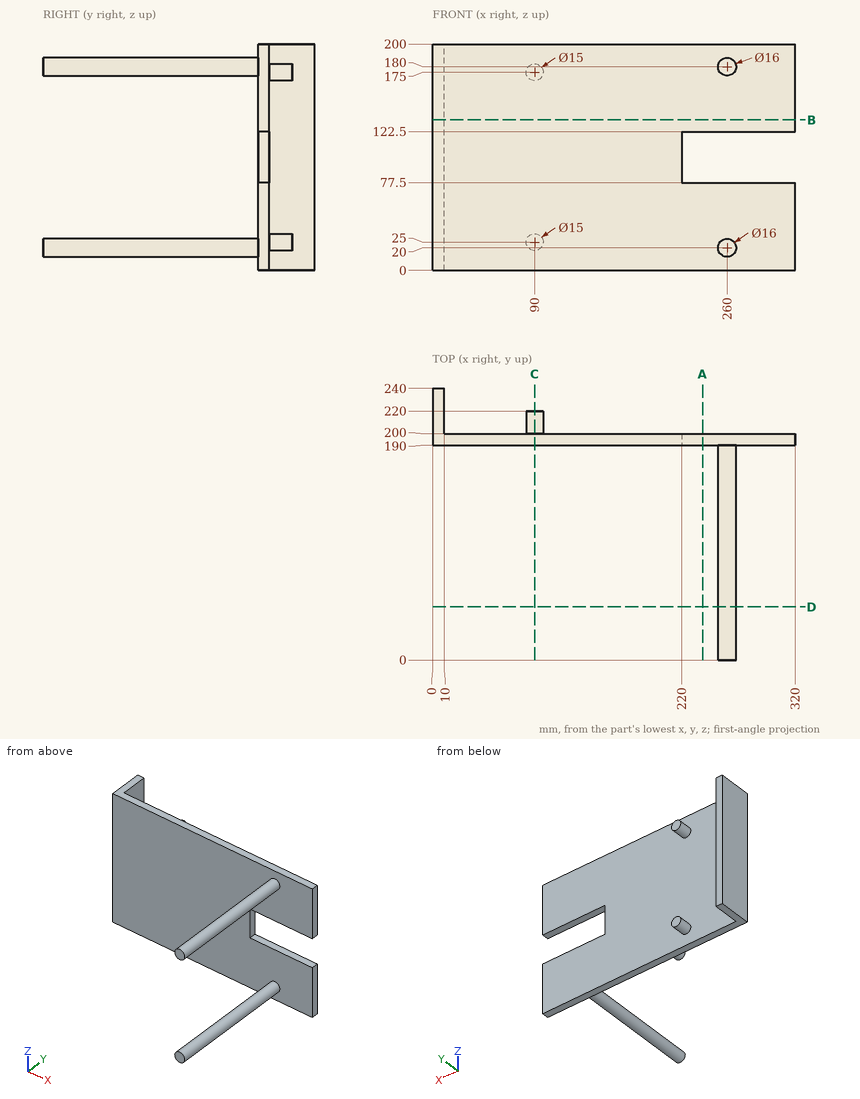
Can you work these out from the drawing? Everything is in mm from the part's minimum corner. Give positions to 0.01 mm unless a question says otherwise; leave off trailing zeros. Order: outer loops, then holes, each group sorted by start corner. A loop starts at its lowest first (then second) coordinate and runs counter-clockwise, first axis right, second up. Notation, with made-up numbers: M 82,32 L 137,32 A25 cw 137,71 Z; hole C 39,54.25 d10. An arc over 180 degrees is marked long. Use a Markdown table: item, result. Add a question column.
Item 1: Suppose I cut it at D-D (y = 47). List the corners of the cut face in (x, z) for me, then the cut area to 3 significant figures.
Item 2: Suppose I cut it at A-A (x = 238.5). List the corners of the cut face in (y, z) for me, then the cut area to 3 significant figures.
Item 3: Suppose I cut it at B-B (z = 133). List the corners of the cut face in (x, y) for me.
Item 4: Suppose I cut it at C-C (x = 90). List the corners of the cut face in (y, z) for me.
Item 5: Will these pins go through, and if not, where does the flat tip stop? pin 1 (1.5 mm diameter, centred on x = 136, z = 87, fed in from -Y); pin 2 (4.5 mm diameter, centred on x = 90.5, z = 26.5, fed in from +Y); pin 3 (12 mm diameter, centred on y = 213.5, z = 127.5, fed in from +X); pin 4 (8 mm diameter, centred on x = 251, y = 197.5, fed in from -Z).
Item 6: If I drill on L1, parallel to X at y = 223, z = 174.5; L2, parallel to Y at x = 188, z = 126; L3, parallel to X at y = 55, z = 21.5, over which ranges is the centre line in solid material (lowest first)? Write a range as [from, to].
Answer sheet:
| question | item | result |
|---|---|---|
| 1 | outline | C 260,20 d16; C 260,180 d16 |
| 1 | area | 402 mm² |
| 2 | outline | M 190,0 L 200,0 L 200,77.5 L 190,77.5 Z; M 190,122.5 L 200,122.5 L 200,200 L 190,200 Z |
| 2 | area | 1,550 mm² |
| 3 | outline | M 0,190 L 320,190 L 320,200 L 10,200 L 10,240 L 0,240 Z |
| 4 | outline | M 190,0 L 200,0 L 200,17.5 L 220,17.5 L 220,32.5 L 200,32.5 L 200,167.5 L 220,167.5 L 220,182.5 L 200,182.5 L 200,200 L 190,200 Z |
| 5 | pin 1 | stops at y = 190 |
| 5 | pin 2 | stops at y = 220 |
| 5 | pin 3 | stops at x = 10 |
| 5 | pin 4 | stops at z = 0 |
| 6 | L1 | x = [0, 10] |
| 6 | L2 | y = [190, 200] |
| 6 | L3 | x = [252.14, 267.86] |
